Build history of the part. All positions in model axes, mm. A direction names the side the tool comes from. Round coordinates to 2 decimals unless told otherwise and drop trailing zeros. Order: outer loops, then holes, each group sorted by start corner. A loop starts at its lowest first (then second) coordinate and runs counter-clockwise, first axis right, second up. Notation, with made-up numbers: (70.25, 54.5) -> (122.25, 54.5) arc R24 cw to (122.25, 69.5) -> close; hole circle Ø8 at (-23, 60.25). An arc over 180 degrees is marked (long way). Answer as CSV lines item,"result". Start each with the question number.
```python
from build123d import *

# Parameters (mm, degrees)
SKETCH1_W           = 14.605
SKETCH1_H           = 46.482
SKETCH1_R           = 1.905
BOSS_EXTRUDE1_DEPTH = 44.45
SKETCH2_W           = 4.445
SKETCH2_H           = 33.02
CUT_EXTRUDE1_DEPTH  = 38.1
SKETCH3_W           = 42.545
SKETCH3_H           = 25.4
CUT_EXTRUDE2_DEPTH  = 12.065
CUT_EXTRUDE3_DEPTH  = 40.64
FILLET1_R           = 2.54
FILLET2_R           = 1.016
CHAMFER1_SIZE       = 7.62


with BuildPart() as part:
    # Sketch1 → Boss-Extrude1 (new body)
    with BuildSketch(Plane.XY):
        with Locations((7.3025, 23.241)):
            Rectangle(SKETCH1_W, SKETCH1_H)
        with Locations((4.191, 42.291)):
            Circle(SKETCH1_R, mode=Mode.SUBTRACT)
        with Locations((4.191, 4.191)):
            Circle(SKETCH1_R, mode=Mode.SUBTRACT)
    extrude(amount=BOSS_EXTRUDE1_DEPTH)

    # Sketch2 → Cut-Extrude1 (cut)
    with BuildSketch(Plane.XY.offset(44.45)):
        with Locations((11.1125, 23.241)):
            Rectangle(SKETCH2_W, SKETCH2_H)
    extrude(amount=-CUT_EXTRUDE1_DEPTH, mode=Mode.SUBTRACT)

    # Sketch3 → Cut-Extrude2 (cut)
    with BuildSketch(Plane.ZY.offset(-13.335)):
        with Locations((21.2725, 23.241)):
            Rectangle(SKETCH3_W, SKETCH3_H)
    extrude(amount=CUT_EXTRUDE2_DEPTH, mode=Mode.SUBTRACT)

    # Sketch4 → Cut-Extrude3 (cut)
    with BuildSketch(Plane.XY.offset(44.45)):
        with BuildLine():
            Line((4.191, 38.1), (0, 38.1))
            Line((0, 38.1), (0, 46.482))
            Line((0, 46.482), (8.382, 46.482))
            Line((8.382, 46.482), (8.382, 42.291))
            ThreePointArc((8.382, 42.291), (7.15448452, 39.32751548), (4.191, 38.1))
        make_face()
        with BuildLine():
            Line((4.191, 8.382), (0, 8.382))
            Line((0, 8.382), (0, 0))
            Line((0, 0), (8.382, 0))
            Line((8.382, 0), (8.382, 4.191))
            ThreePointArc((8.382, 4.191), (7.15448452, 7.15448452), (4.191, 8.382))
        make_face()
    extrude(amount=-CUT_EXTRUDE3_DEPTH, mode=Mode.SUBTRACT)

    # Fillet1
    fillet1_edges = [part.edges().sort_by_distance(p)[0] for p in [
        (0, 46.482, 1.905),
        (8.382, 46.482, 24.13),
        (0, 38.1, 24.13),
        (14.605, 46.482, 22.225),
        (0, 0, 1.905),
        (14.605, 0, 22.225),
        (8.382, 0, 24.13),
        (0, 8.382, 24.13),
    ]]
    fillet(fillet1_edges, radius=FILLET1_R)

    # Fillet2
    fillet2_edges = [part.edges().sort_by_distance(p)[0] for p in [
        (3.3655, 38.1, 44.45),
        (0, 23.241, 44.45),
        (13.861051224, 45.738051224, 44.45),
        (13.861051224, 0.743948776, 44.45),
        (9.125948776, 0.743948776, 44.45),
        (0.743948776, 9.125948776, 44.45),
        (0.743948776, 37.356051224, 44.45),
        (9.125948776, 45.738051224, 44.45),
        (7.15448452, 39.32751548, 44.45),
        (8.382, 43.1165, 44.45),
        (7.15448452, 7.15448452, 44.45),
        (3.3655, 8.382, 44.45),
        (11.4935, 46.482, 44.45),
        (8.382, 3.3655, 44.45),
        (11.4935, 0, 44.45),
        (14.605, 23.241, 44.45),
    ]]
    fillet(fillet2_edges, radius=FILLET2_R)

    # Chamfer1
    chamfer1_edges = [part.edges().sort_by_distance(p)[0] for p in [
        (1.27, 23.241, 42.545),
    ]]
    chamfer(chamfer1_edges, length=CHAMFER1_SIZE - 0.0001)  # a hair under: the kernel refuses the full size


solid = part.part
```
Q1. Probe L1, parallel to X at y = 18, z = 8 (3 decimals); L2, parallel to X at y = 34.5, z = 43.5 (3 decimals); L3, parallel to Y at x = 4.25, z = 10. List the from-to ranges inside material, lowest first.
Q2. Flat gauge pins, fed straight in: pin 1 Ø1.8 at (x, z) = (3, 20) entering from +Y; pin 2 Ø3 at (y, z) = (8.5, 13) entering from -X; pin 3 Ø6 at (x, z) = (7, 24) entering from -Y; pin 4 Ø6 at (x, y) = (7.5, 39.5) entering from +Z. Where does each tip first touch, or does it go through?
Q3. Slice it at A-A, the plane x = 11.5. Write the cut outline in (y, z).
Q4. Which spindle directions (+Z, -Z, +X, -X, +Y, -Y) get a long thin tool onto all of the face, cutting with end or side? Do faces 4 (the face through (6, 10.541, 16)), 5 (the face through (3.354, 37.81, 44.144)), 6 (the face through (11, 38, 6.35)), 7 (the face through (3, 8.382, 24)). Say none if no direction does.
Q5. Slice it at C-C, the plane z = 19.5. Write the cut outline in (x, y) (3 decimals), plus the area to 3 significant figures.
Q6. Two-plate mould, pull along X, no slides. Class faces 1 (the face through (8.89, 10, 28)), 2 (the face through (6, 24, 44.45)), 3 (the face through (7.187, 39.36, 23.899)): +X half, -X half, draft (parallel to the pull), parting line (faces both ways), or undercut.
Q7. Slice it at D-D, the plane x = 5.5. Count the separate pieces of the cut face and the enclosed holes in it, plus the area to 3 significant figures.
Solutions:
1,L1,"x = 0 to 1.27, 13.335 to 14.605"
1,L2,"x = 0.002 to 8.89, 13.335 to 14.603"
1,L3,"y = 8.38 to 10.54, 35.94 to 38.1"
2,pin 1,"stops at y = 38.1"
2,pin 2,"stops at x = 0.17"
2,pin 3,"stops at y = 0.17"
2,pin 4,"stops at z = 44.45"
3,outline,"(0, 0) -> (10.54, 0) -> (10.54, 6.35) -> (6.73, 6.35) -> (6.73, 44.45) -> (1.02, 44.45) arc R1.02 ccw to (0, 43.43) -> close; (35.94, 0) -> (46.48, 0) -> (46.48, 43.43) arc R1.02 ccw to (45.47, 44.45) -> (39.75, 44.45) -> (39.75, 6.35) -> (35.94, 6.35) -> close"
4,face 4,"-Z"
4,face 5,"+Z, -X, +Y"
4,face 6,"+Z"
4,face 7,"+Z, -X, -Y"
5,outline,"(0, 10.922) arc R2.54 ccw to (2.54, 8.382) -> (4.191, 8.382) arc R4.191 cw to (8.382, 4.191) -> (8.382, 2.54) arc R2.54 ccw to (10.922, 0) -> (12.065, 0) arc R2.54 ccw to (14.605, 2.54) -> (14.605, 43.942) arc R2.54 ccw to (12.065, 46.482) -> (10.922, 46.482) arc R2.54 ccw to (8.382, 43.942) -> (8.382, 42.291) arc R4.191 cw to (4.191, 38.1) -> (2.54, 38.1) arc R2.54 ccw to (0, 35.56) -> close; hole (1.27, 10.541) -> (8.89, 10.541) -> (8.89, 6.731) -> (13.335, 6.731) -> (13.335, 39.751) -> (8.89, 39.751) -> (8.89, 35.941) -> (1.27, 35.941) -> close"
5,area,"197 mm2"
6,face 1,"undercut"
6,face 2,"draft"
6,face 3,"-X half"
7,separate pieces,"3"
7,enclosed holes,"0"
7,area,"386 mm2"
